```python
from build123d import *

# Parameters (mm, degrees)
F1_DEPTH       = 12.7
F3_D           = 3.81
F3_CSINK_D     = 5.08
F3_CSINK_ANGLE = 45


with BuildPart() as f1:
    # F0 (on Front) → F1 (new body, symmetric)
    with BuildSketch(Plane.XZ):
        with BuildLine():
            Line((-38.1, 4.7625), (-3.175, 4.7625))
            ThreePointArc((-3.175, 4.7625), (-0.929936, 5.692436), (0, 7.9375))
            Line((0, 7.9375), (0, 42.8625))
            Line((0, 42.8625), (-3.175, 42.8625))
            Line((-3.175, 42.8625), (-3.175, 9.525))
            ThreePointArc((-3.175, 9.525), (-3.639968, 8.402468), (-4.7625, 7.9375))
            Line((-4.7625, 7.9375), (-38.1, 7.9375))
            Line((-38.1, 7.9375), (-38.1, 4.7625))
        make_face()
    extrude(amount=F1_DEPTH, both=True)

    # F3 (through all)
    with Locations(Plane.YZ):
        with Locations((-9.201728, 39.201986)):
            CounterSinkHole(F3_D / 2, F3_CSINK_D / 2, counter_sink_angle=F3_CSINK_ANGLE)


solid = f1.part
```
Source: CAD feature listing. Evaluate the final solid. Frame: model axes, mm. A direction names the side the tool comes from. Coordinates: 2 decimals unless noted, no trailing zeros. Loops run counter-clockwise (first coordinate to the right, second up) from the corner with the lowest first, then second, coordinate; pieces in that order, holes last. Notation, with made-up numbers: M -37,70.5 L 15,70.5 A17 ccw 15,78.5 Z; hole C 88,42.5 d4. An arc over 180 degrees is marked long. Use a Markdown table: item, result. Add a question column.
Q1. Section query C-C, the plane x = -24.5. Return loops of the section in (y, z).
Q2. Draft query along Z for faces 1 (the flat face through (-11, 12.7, 7)), 2 (the cylindrical face through (-2.366, -10.226, 40.808)), 3 (the flat face through (-21, 0, 7.938)). Return one class per face: pulls with the +Z half, pulls with the -Z half, needs draft (parallel to the pull), parting line crosses it, or undercut.
Q3. Access query for faces 4 (the flat face through (-3.175, 0, 26)), 5 (the flat face through (-2, 0, 42.862)). Directions: +Z, -Z, +X, -X, +Y, -Y. A direction counts if a zero-diameter tool reaches every point of the face in a straight line with its end or side. Return the directions, or none.
Q4. First-contact query: pin 1 (6 mm diameter, centred on x = -20, y = 8.5, fed in from +Z); pin 2 (5 mm diameter, centred on y = -9.2, z = 39.2, fed in from -X) (3 decimals). Flat tips, straight axial feed; report the tip coordinate or a pass-through.
Q5. Section query B-B, the plane z = 32. Return loops of the section in (x, y) (3 decimals).
Q6. Material intervals for L1, parallel to X at y = -5, z = 30 (3 decimals); L2, parallel to Z at x = -21.5, y = -8.5; L3, parallel to Z at x = -2.5, y = -10.75, sorted ascending.
Result:
| question | item | result |
|---|---|---|
| 1 | outline | M -12.7,4.76 L 12.7,4.76 L 12.7,7.94 L -12.7,7.94 Z |
| 2 | face 1 | needs draft |
| 2 | face 2 | undercut |
| 2 | face 3 | pulls with the +Z half |
| 3 | face 4 | +Z, -X, +Y, -Y |
| 3 | face 5 | +Z, +X, -X, +Y, -Y |
| 4 | pin 1 | stops at z = 7.94 |
| 4 | pin 2 | stops at x = -3.175 |
| 5 | outline | M -3.175,-12.7 L 0,-12.7 L 0,12.7 L -3.175,12.7 Z |
| 6 | L1 | x = -3.175 to 0 |
| 6 | L2 | z = 4.76 to 7.94 |
| 6 | L3 | z = 4.84 to 38.09, 40.31 to 42.86 |
